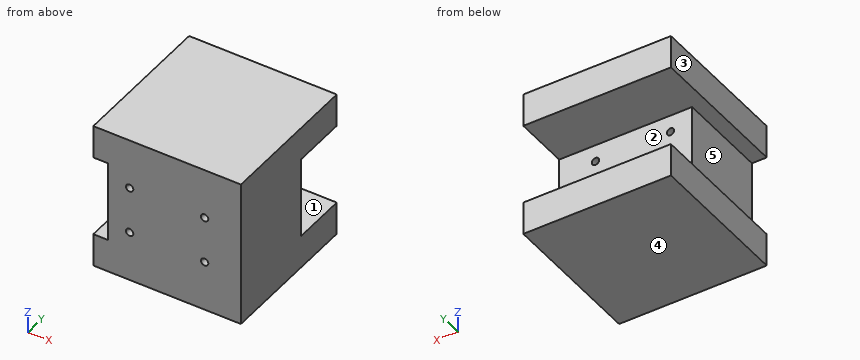
Autodesk Inventor part; units mm, degrees
ref_plane "YZ Plane" through (0, 0, 0) normal (1, 0, 0) x (0, 1, 0)
ref_plane "XZ Plane" through (0, 0, 0) normal (0, 1, 0) x (-1, 0, 0)
ref_plane "XY Plane" through (0, 0, 0) normal (0, 0, 1) x (1, 0, 0)
sketch "Sketch1" plane through (0, 0, 0) normal (0, 1, 0) x (-1, 0, 0)
  line L0 (-20, -20) -> (20, -20)
  line L1 (20, -20) -> (20, 20)
  line L2 (20, 20) -> (-20, 20)
  line L3 (-20, 20) -> (-20, -20)
  line L4 (-20, -20) -> (20, 20) construction
  line L5 (20, -20) -> (-20, 20) construction
  point P0 (0, 0)
  dimension "d0" = 40
extrude "Extrusion1" add sketch "Sketch1" along normal mid plane 40
sketch "Sketch2" plane through (0, 20, 0) normal (0, 1, 0) x (1, 0, 0)
  line L0 (-20, 20) -> (-20, -20)
  line L1 (20, -11) -> (-20, -11)
  line L2 (-20, -11) -> (-20, 11)
  line L3 (-20, 11) -> (20, 11)
  line L4 (20, 11) -> (20, -11)
  line L5 (20, -11) -> (-20, 11) construction
  line L6 (-20, -11) -> (20, 11) construction
  line L7 (-24, -11) -> (-16, -11)
  line L8 (-16, -11) -> (-16, 11)
  line L9 (-16, 11) -> (-24, 11)
  line L10 (-24, 11) -> (-24, -11)
  line L11 (-24, -11) -> (-16, 11) construction
  line L12 (-16, -11) -> (-24, 11) construction
  line L13 (-10.16, 6.35) -> (10.16, 6.35) construction
  line L14 (10.16, 6.35) -> (10.16, -6.35) construction
  line L15 (10.16, -6.35) -> (-10.16, -6.35) construction
  line L16 (-10.16, -6.35) -> (-10.16, 6.35) construction
  line L17 (-10.16, 6.35) -> (10.16, -6.35) construction
  line L18 (10.16, 6.35) -> (-10.16, -6.35) construction
  circle A0 centre (10.16, -6.35) radius 1
  circle A1 centre (-10.16, -6.35) radius 1
  circle A2 centre (-10.16, 6.35) radius 1
  circle A3 centre (10.16, 6.35) radius 1
  point P0 (0, 0)
  point P1 (-20, -11)
  point P2 (-20, 0)
  point P3 (-20, -11)
  point P4 (-16, -11)
  dimension "d3" = 22
  dimension "d6" = 8
  dimension "d9" = 12.7
  dimension "d10" = 20.32
  dimension "d11" = 2
extrude "Extrusion2" cut sketch "Sketch2" against normal blind 15 contours L3 L8 L1 L0 | L3 L4 L1 L8 | A0 | A1 | A2 | A3
extrude "Extrusion3" cut sketch "Sketch2" against normal through all contours L3 L8 L1 L0 | L0 L7 L10 L9
extrude "Extrusion4" cut sketch "Sketch2" against normal through all contours A0 | A1 | A2 | A3
properties part number "IMU_Calibration_Cube"
Input: part model. Units: mm. Frame: model coordinates. Face numbers are marked on the shaded views. A direction names the side the tool comes from. Coordinates: 2 decimals unless noted, no trailing zeros. Loops run counter-clockwise (first coordinate to the right, second up) from the corner with the lowest first, then second, coordinate; pieces in that order, holes last. Notation, with made-up numbers: (25, 89.25) - (71, 89.25) arc R15 cw to (71, 108.25) - close; hole circle Ø1 at (56, -18). An arc over 180 degrees is marked (long way). Answer in a Markdown table with one row per item.
(1) Pin query (flat end, axial travel): P1, Ø3, axis at x = -10.16, z = -6.35, coming from the -Y side; P2, Ø4, axis at y = 6, z = 7, coming from the -X side; P3, Ø2.5, axis at x = 10.16, z = 6.35, coming from the +Y side. Return the tip coordinate at first contact, or that it passes through.
Model answer:
| item | result |
|---|---|
| P1 | stops at y = -20 |
| P2 | stops at x = -16 |
| P3 | stops at y = 5 |
(2) Material intervals for L1, parallel to X at y = -4, z = 6.35; L2, parallel to Z at x = -10, y = -2.5; L3, parallel to Z at x = -17.5, y = -2, sorted ascending. Write a range as from..to.
Model answer:
| item | result |
|---|---|
| L1 | x = -16..-11.16, -9.16..9.16, 11.16..20 |
| L2 | z = -20..-7.34, -5.36..5.36, 7.34..20 |
| L3 | z = -20..-11, 11..20 |
(3) Cut plane D-D on y = 13. Output: boundary loops of the cut face in (x, z), plus the area to 3 significant figures.
Model answer:
| item | result |
|---|---|
| outline | (-20, -20) - (20, -20) - (20, -11) - (-20, -11) - close; (-20, 11) - (20, 11) - (20, 20) - (-20, 20) - close |
| area | 720 mm² |
(4) Cut plane A-A on x = -10.16. Output: boundary loops of the cut face in (y, z).
Model answer:
| item | result |
|---|---|
| outline | (-20, -20) - (20, -20) - (20, -11) - (5, -11) - (5, -7.35) - (-20, -7.35) - close; (-20, -5.35) - (5, -5.35) - (5, 5.35) - (-20, 5.35) - close; (-20, 7.35) - (5, 7.35) - (5, 11) - (20, 11) - (20, 20) - (-20, 20) - close |
(5) Cut plane B-B on z = 6.35. Output: boundary loops of the cut face in (x, y), plus the area to 3 significant figures.
Model answer:
| item | result |
|---|---|
| outline | (-16, -20) - (-11.16, -20) - (-11.16, 5) - (-16, 5) - close; (-9.16, -20) - (9.16, -20) - (9.16, 5) - (-9.16, 5) - close; (11.16, -20) - (20, -20) - (20, 5) - (11.16, 5) - close |
| area | 800 mm² |
(6) Cut plane C-C on y = 1. Output: boundary loops of the cut face in (x, z).
Model answer:
| item | result |
|---|---|
| outline | (-20, -20) - (20, -20) - (20, 20) - (-20, 20) - (-20, 11) - (-16, 11) - (-16, -11) - (-20, -11) - close; hole circle Ø2 at (-10.16, -6.35); hole circle Ø2 at (-10.16, 6.35); hole circle Ø2 at (10.16, -6.35); hole circle Ø2 at (10.16, 6.35) |
(7) Set-up query: the marked faces 1, 2, 3, 4 and 5. Return all of +Z, -Z, +X, -X, +Y, -Y with unobstructed straight access to the full face (end or side cutting, diameter ignored); none if empty.
Model answer:
| item | result |
|---|---|
| face 1 | -X, +Y |
| face 2 | +X, -X, +Y |
| face 3 | +Z, -Z, -X, +Y, -Y |
| face 4 | -Z, +X, -X, +Y, -Y |
| face 5 | -X, +Y, -Y |
